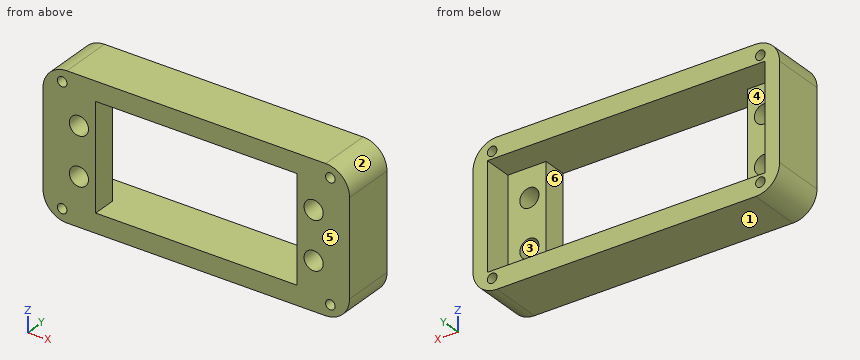
from build123d import *

# Parameters (mm, degrees)
SKETCH2_W           = 64
SKETCH2_H           = 30
BOSS_EXTRUDE1_DEPTH = 64
CUT_EXTRUDE1_REACH  = 97.352
SKETCH3_W           = 42
SKETCH3_H           = 22
CUT_EXTRUDE2_REACH  = 97.352
SKETCH4_R           = 2
SKETCH5_W           = 64
SKETCH5_H           = 30
SKETCH5_W_2         = 58
SKETCH5_H_2         = 22
BOSS_EXTRUDE2_DEPTH = 12
CUT_EXTRUDE3_REACH  = 105.788
SKETCH6_R           = 1
FILLET1_R           = 5
CUT_EXTRUDE4_DEPTH  = 59
CUT_EXTRUDE7_DEPTH  = 6


with BuildPart() as part:
    # Sketch2 → Boss-Extrude1 (new body)
    with BuildSketch(Plane(origin=(0, 0, 0), x_dir=(1, 0, 0), z_dir=(0, 1, 0))):
        with Locations((32, 15)):
            Rectangle(SKETCH2_W, SKETCH2_H)
    extrude(amount=BOSS_EXTRUDE1_DEPTH)

    # Sketch3 → Cut-Extrude1 (cut, up to next)
    with BuildSketch(Plane(origin=(0, 64, 0), x_dir=(1, 0, 0), z_dir=(0, 1, 0)), mode=Mode.PRIVATE) as cut_extrude1_sk1:
        with Locations((32, 15)):
            Rectangle(SKETCH3_W, SKETCH3_H)
    cut_extrude1_tool1 = extrude(cut_extrude1_sk1.sketch, amount=-CUT_EXTRUDE1_REACH, mode=Mode.PRIVATE) & part.part
    add(cut_extrude1_tool1.solids().sort_by_distance((32, 64, -15))[0], mode=Mode.SUBTRACT)

    # Sketch4 → Cut-Extrude2 (cut, up to next)
    with BuildSketch(Plane(origin=(0, 64, 0), x_dir=(1, 0, 0), z_dir=(0, 1, 0)), mode=Mode.PRIVATE) as cut_extrude2_sk1:
        with Locations(Location((7.5, 20, 0), (0, 0, 270))):
            Circle(SKETCH4_R)
    cut_extrude2_tool1 = extrude(cut_extrude2_sk1.sketch, amount=-CUT_EXTRUDE2_REACH, mode=Mode.PRIVATE) & part.part
    # Sketch4 → Cut-Extrude2 (cut, up to next)
    with BuildSketch(Plane(origin=(0, 64, 0), x_dir=(1, 0, 0), z_dir=(0, 1, 0)), mode=Mode.PRIVATE) as cut_extrude2_sk2:
        with Locations(Location((7.5, 10, 0), (0, 0, 90))):
            Circle(SKETCH4_R)
    cut_extrude2_tool2 = extrude(cut_extrude2_sk2.sketch, amount=-CUT_EXTRUDE2_REACH, mode=Mode.PRIVATE) & part.part
    # Sketch4 → Cut-Extrude2 (cut, up to next)
    with BuildSketch(Plane(origin=(0, 64, 0), x_dir=(1, 0, 0), z_dir=(0, 1, 0)), mode=Mode.PRIVATE) as cut_extrude2_sk3:
        with Locations(Location((56.5, 10, 0), (0, 0, 270))):
            Circle(SKETCH4_R)
    cut_extrude2_tool3 = extrude(cut_extrude2_sk3.sketch, amount=-CUT_EXTRUDE2_REACH, mode=Mode.PRIVATE) & part.part
    # Sketch4 → Cut-Extrude2 (cut, up to next)
    with BuildSketch(Plane(origin=(0, 64, 0), x_dir=(1, 0, 0), z_dir=(0, 1, 0)), mode=Mode.PRIVATE) as cut_extrude2_sk4:
        with Locations(Location((56.5, 20, 0), (0, 0, 90))):
            Circle(SKETCH4_R)
    cut_extrude2_tool4 = extrude(cut_extrude2_sk4.sketch, amount=-CUT_EXTRUDE2_REACH, mode=Mode.PRIVATE) & part.part
    add(cut_extrude2_tool1.solids().sort_by_distance((7.5, 64, -20))[0], mode=Mode.SUBTRACT)
    add(cut_extrude2_tool2.solids().sort_by_distance((7.5, 64, -10))[0], mode=Mode.SUBTRACT)
    add(cut_extrude2_tool3.solids().sort_by_distance((56.5, 64, -10))[0], mode=Mode.SUBTRACT)
    add(cut_extrude2_tool4.solids().sort_by_distance((56.5, 64, -20))[0], mode=Mode.SUBTRACT)

    # Sketch5 → Boss-Extrude2 (add)
    with BuildSketch(Plane(origin=(0, 64, 0), x_dir=(1, 0, 0), z_dir=(0, 1, 0))):
        with Locations((32, 15)):
            Rectangle(SKETCH5_W, SKETCH5_H)
        with Locations((32, 15)):
            Rectangle(SKETCH5_W_2, SKETCH5_H_2, mode=Mode.SUBTRACT)
    extrude(amount=BOSS_EXTRUDE2_DEPTH)

    # Sketch6 → Cut-Extrude3 (cut, up to next)
    with BuildSketch(Plane(origin=(0, 76, 0), x_dir=(1, 0, 0), z_dir=(0, 1, 0)), mode=Mode.PRIVATE) as cut_extrude3_sk1:
        with Locations(Location((4, 27.5, 0), (0, 0, 270))):
            Circle(SKETCH6_R)
    cut_extrude3_tool1 = extrude(cut_extrude3_sk1.sketch, amount=-CUT_EXTRUDE3_REACH, mode=Mode.PRIVATE) & part.part
    # Sketch6 → Cut-Extrude3 (cut, up to next)
    with BuildSketch(Plane(origin=(0, 76, 0), x_dir=(1, 0, 0), z_dir=(0, 1, 0)), mode=Mode.PRIVATE) as cut_extrude3_sk2:
        with Locations(Location((4, 2.5, 0), (0, 0, 90))):
            Circle(SKETCH6_R)
    cut_extrude3_tool2 = extrude(cut_extrude3_sk2.sketch, amount=-CUT_EXTRUDE3_REACH, mode=Mode.PRIVATE) & part.part
    # Sketch6 → Cut-Extrude3 (cut, up to next)
    with BuildSketch(Plane(origin=(0, 76, 0), x_dir=(1, 0, 0), z_dir=(0, 1, 0)), mode=Mode.PRIVATE) as cut_extrude3_sk3:
        with Locations(Location((60, 2.5, 0), (0, 0, 270))):
            Circle(SKETCH6_R)
    cut_extrude3_tool3 = extrude(cut_extrude3_sk3.sketch, amount=-CUT_EXTRUDE3_REACH, mode=Mode.PRIVATE) & part.part
    # Sketch6 → Cut-Extrude3 (cut, up to next)
    with BuildSketch(Plane(origin=(0, 76, 0), x_dir=(1, 0, 0), z_dir=(0, 1, 0)), mode=Mode.PRIVATE) as cut_extrude3_sk4:
        with Locations(Location((60, 27.5, 0), (0, 0, 90))):
            Circle(SKETCH6_R)
    cut_extrude3_tool4 = extrude(cut_extrude3_sk4.sketch, amount=-CUT_EXTRUDE3_REACH, mode=Mode.PRIVATE) & part.part
    add(cut_extrude3_tool1.solids().sort_by_distance((4, 76, -27.5))[0], mode=Mode.SUBTRACT)
    add(cut_extrude3_tool2.solids().sort_by_distance((4, 76, -2.5))[0], mode=Mode.SUBTRACT)
    add(cut_extrude3_tool3.solids().sort_by_distance((60, 76, -2.5))[0], mode=Mode.SUBTRACT)
    add(cut_extrude3_tool4.solids().sort_by_distance((60, 76, -27.5))[0], mode=Mode.SUBTRACT)

    # Fillet1
    fillet1_edges = [part.edges().sort_by_distance(p)[0] for p in [
        (0, 38, -30),
        (64, 38, -30),
        (64, 38, 0),
        (0, 38, 0),
    ]]
    fillet(fillet1_edges, radius=FILLET1_R)

    # Sketch7 → Cut-Extrude4 (cut)
    with BuildSketch(Plane.XZ):
        with BuildLine():
            Line((5, -30), (59, -30))
            ThreePointArc((59, -30), (62.535533906, -28.535533906), (64, -25))
            Line((64, -25), (64, -5))
            ThreePointArc((64, -5), (62.535533906, -1.464466094), (59, 0))
            Line((59, 0), (5, 0))
            ThreePointArc((5, 0), (1.464466094, -1.464466094), (0, -5))
            Line((0, -5), (0, -25))
            ThreePointArc((0, -25), (1.464466094, -28.535533906), (5, -30))
        make_face()
    extrude(amount=-CUT_EXTRUDE4_DEPTH, mode=Mode.SUBTRACT)

    # Sketch10 → Cut-Extrude7 (cut)
    with BuildSketch(Plane(origin=(0, 76, 0), x_dir=(1, 0, 0), z_dir=(0, 1, 0))):
        with BuildLine():
            Line((64, 5), (64, 25))
            ThreePointArc((64, 25), (62.535533906, 28.535533906), (59, 30))
            Line((59, 30), (5, 30))
            ThreePointArc((5, 30), (1.464466094, 28.535533906), (0, 25))
            Line((0, 25), (0, 5))
            ThreePointArc((0, 5), (1.464466094, 1.464466094), (5, 0))
            Line((5, 0), (59, 0))
            ThreePointArc((59, 0), (62.535533906, 1.464466094), (64, 5))
        make_face()
    extrude(amount=-CUT_EXTRUDE7_DEPTH, mode=Mode.SUBTRACT)


solid = part.part
The listing builds one solid part. Answer for the finished solid, in the listing's coordinates (mm). Face numbers are marked on the shaded views. A direction names the side the tool comes from. Give positions to 0.01 mm unless a question says otherwise; leave off trailing zeros. Order: outer loops, then holes, each group sorted by start corner. A loop starts at its lowest first (then second) coordinate and runs counter-clockwise, first axis right, second up. Notation, with made-up numbers: (55.5, -17) -> (83.5, -17) arc R21 cw to (83.5, -5) -> close; hole circle Ø2 at (73, 17). An arc over 180 degrees is marked (long way). Put each result on its own line as item: value.
Item 1: Straight lines are drawn through the part: line 1 (X direction, y = 67.25, z = -19); line 2 (Z direction, x = 13, y = 64); line 3 (X direction, y = 62.15, z = -10). For each, find the intervals that lie inside material, in ascending order.
Established:
line 1: x = 0 to 3, 61 to 64
line 2: z = -30 to -26, -4 to 0
line 3: x = 0 to 5.5, 9.5 to 11, 53 to 54.5, 58.5 to 64
Item 2: A cutting plane is placed at C-C on x = 56.5. Give the vertices of the cut face in (y, z), plus the area to 3 significant figures.
Established:
outline: (59, -30) -> (70, -30) -> (70, -26) -> (64, -26) -> (64, -22) -> (59, -22) -> close; (59, -18) -> (64, -18) -> (64, -12) -> (59, -12) -> close; (59, -8) -> (64, -8) -> (64, -4) -> (70, -4) -> (70, 0) -> (59, 0) -> close
area: 158 mm^2
Item 3: For a pull along X with two mould halves and no side action, classify the marked faces 1, 2 and 3 as released by +X, released by -X, zero draft, split by the parting line, or undercut.
Established:
face 1: zero draft
face 2: released by +X
face 3: undercut
Item 4: A cutting plane is placed at B-B on y = 68.75. Give the vertices of the cut face in (x, z).
Established:
outline: (0, -25) arc R5 ccw to (5, -30) -> (59, -30) arc R5 ccw to (64, -25) -> (64, -5) arc R5 ccw to (59, 0) -> (5, 0) arc R5 ccw to (0, -5) -> close; hole circle Ø2 at (4, -27.5); hole (3, -26) -> (61, -26) -> (61, -4) -> (3, -4) -> close; hole circle Ø2 at (4, -2.5); hole circle Ø2 at (60, -27.5); hole circle Ø2 at (60, -2.5)
Item 5: For the marked faces 4, 5 and 6, determine the directions among +Z, -Z, +X, -X, +Y, -Y from which every point of the face is accessible in a straight line to the end or side of a thin tool.
Established:
face 4: +Y
face 5: +Z, -Z, +X, -X, -Y
face 6: +Y, -Y
Item 6: Given P1, Ø2.5, axis at x = 7.5, z = -20, coming from the +Y side, flat-ended and moving along its own axis, determine where the tip first touches the part or whether it passes through.
Established:
P1: passes through
Item 7: A cutting plane is placed at D-D on z = -20. Give the vertices of the cut face in (x, y), plus the area to 3 significant figures.
Established:
outline: (0, 59) -> (5.5, 59) -> (5.5, 64) -> (3, 64) -> (3, 70) -> (0, 70) -> close; (9.5, 59) -> (11, 59) -> (11, 64) -> (9.5, 64) -> close; (53, 59) -> (54.5, 59) -> (54.5, 64) -> (53, 64) -> close; (58.5, 59) -> (64, 59) -> (64, 70) -> (61, 70) -> (61, 64) -> (58.5, 64) -> close
area: 106 mm^2
Item 8: A cutting plane is placed at A-A on z = -16.75. Give the vertices of the cut face in (x, y), plus the area to 3 significant figures.
Established:
outline: (0, 59) -> (11, 59) -> (11, 64) -> (3, 64) -> (3, 70) -> (0, 70) -> close; (53, 59) -> (64, 59) -> (64, 70) -> (61, 70) -> (61, 64) -> (53, 64) -> close
area: 146 mm^2
